Geometry: see drawing. Coordinates: mm, zero at the bounding-box minimum. A direction names the side the tool comes from. Round coordinates to 2 decimals unless told otherwise and drop trailing zeros. Write each loop counter-clockwise with the first axis right and the second up, starting at its lowest first coordinate (ties: lowest second). Pieces come first, ordered by that corner, then holes. Notation, with made-up numbers: (13, 43.5) -> (50, 43.5) arc R21 ccw to (50, 72.5) -> close; hole circle Ø8 at (88, 81). An arc over 180 degrees is marked (long way). Write item = value, one per line.
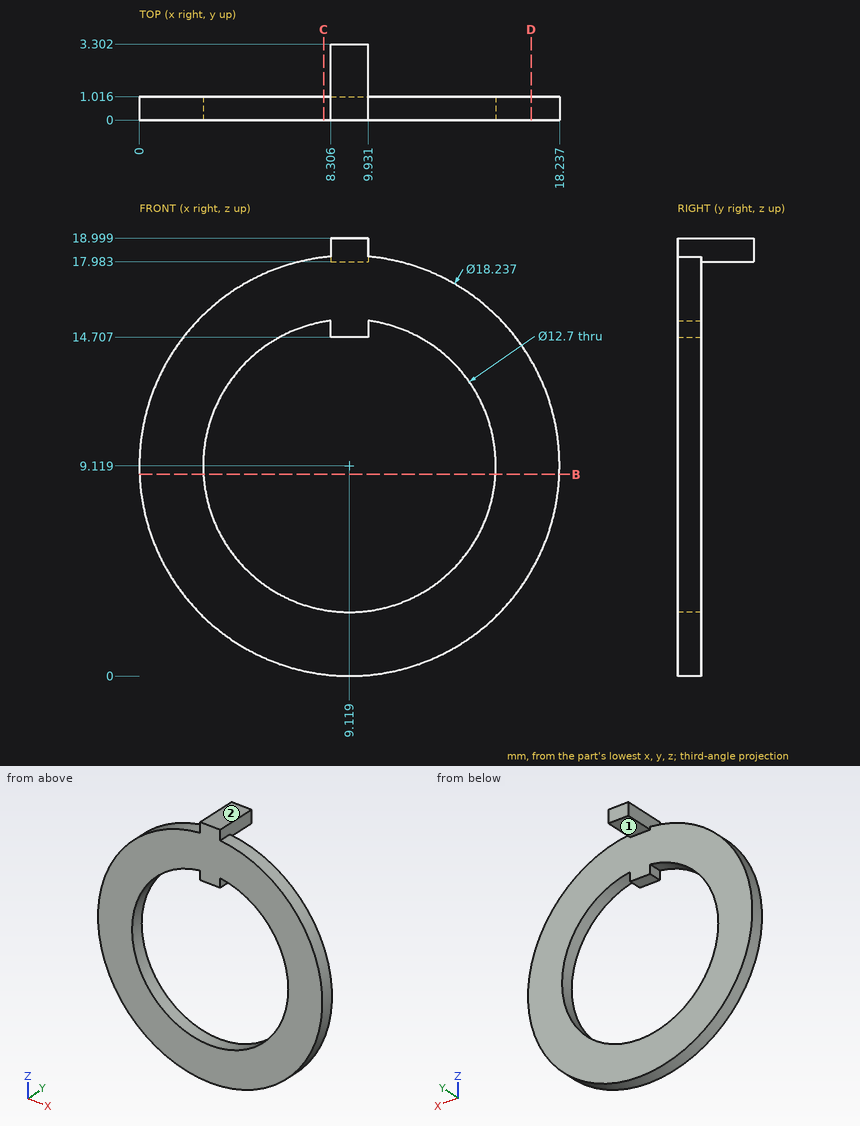
1) Line query: L1, parallel to Y at x = 3, z = 4.5; L2, parallel to X at y = 0.6, z = 12.75 (1 decimal); L3, parallel to X at y = 0.85, z = 13 (1 decimal). Output: solid intervals per line, ascending. Write a range as from..to.
Solutions:
L1 = 0..1.02
L2 = 0.8..3.9, 14.3..17.5
L3 = 0.9..4.1, 14.1..17.4
2) Access query for the marked faces 1 and 2. Directions: +Z, -Z, +X, -X, +Y, -Y. A direction counts if a zero-diameter tool reaches every point of the face in a straight line with its end or side. Return the directions, or none.
Solutions:
face_1 = -Z, +X, -X, +Y
face_2 = +Z, +X, -X, +Y, -Y
3) Cut plane C-C (x = 8). Return the cut outline in (y, z).
Solutions:
outline = (0, 0.07) -> (1.02, 0.07) -> (1.02, 2.87) -> (0, 2.87) -> close; (0, 15.37) -> (1.02, 15.37) -> (1.02, 18.17) -> (0, 18.17) -> close
4) Cut plane B-B (z = 8.75). Return the cut outline in (x, y).
Solutions:
outline = (0.01, 0) -> (2.78, 0) -> (2.78, 1.02) -> (0.01, 1.02) -> close; (15.46, 0) -> (18.23, 0) -> (18.23, 1.02) -> (15.46, 1.02) -> close
5) First-contact query: P1, Ø10, axis at x = 9, z = 5, coming from the +Y side; P2, Ø1.5, axis at x = 3, y = 1, coming from the +Z side; P3, Ø0.5, axis at x = 9, y = 2.5, coming from the -Z side; P4, Ø5, axis at x = 9, z = 11, coming from the +Y side. Flat tips, straight axial feed; report the tip coordinate or a pass-through.
Solutions:
P1 = 1.02
P2 = 16.49
P3 = 17.98
P4 = through
6) Cut plane D-D (x = 17). Return the cut outline in (y, z) (1 decimal).
Solutions:
outline = (0, 4.5) -> (1, 4.5) -> (1, 13.7) -> (0, 13.7) -> close
